Geometry: final body of the model. Coordinates: model frame, mm. A direction names the side the tool comes from. Round coordinates to 2 decimals unless told otherwise and drop trailing zeros. Order: outer loops, then holes, each group sorted by start corner. A loop starts at its lowest first (then second) coordinate and runs counter-clockwise, first axis right, second up. Notation, with made-up numbers: M 70,-36.75 L 121,-36.75 A22 ccw 121,-7.75 Z; hole C -39,85.5 d5. An arc over 180 degrees is marked long. Return JSON: item names as keys, results as strings. Group by question number.
Q1. Ray query, probe 1 along X at (y, z) = (98.5, 4); probe 2 along X at (y, z) = (50.5, 2); probe 3 along Y at (x, z) = (74, 6). Return the intervals inside material, ascending.
Q2. Cut plane A-A on x = 61.5. Output: boundary loops of the cut face in (y, z).
Q3. Contact query for flat-ended pins moving along their axis: pin 1 (5 mm diameter, centred on x = 266, y = 111.5, fed in from -Z); pin 2 (4.5 mm diameter, centred on x = 197, y = 79.5, fed in from +Z); pin 3 (0.6 mm diameter, centred on x = 277, z = 5.5, fed in from -Y). Output: stop coordinate, or through.
Q4. Access query for faces 1 (the face through (11, 90, 4)), 2 (the face through (20, 173, 4)), 3 (the face through (86, 66, 5)). Directions: +Z, -Z, +X, -X, +Y, -Y. A direction counts if a zero-diameter tool reaches every point of the face in a straight line with its end or side. Return the directions, or none.
Q5. Mould query, pull axis X, two halves, no side actions, for faces 4 (the face through (6, 22.5, 4)), 5 (the face through (267.308, 19.363, 3.944)), 6 (the face through (20, 7, 4)), 7 (the face through (76.5, 90, 4)). Classes: released by +X, released by -X, zero draft, split by the parting line, or undercut.
Q6. Cut plane B-B on z = 3. Count the separate pieces of the cut face and the enclosed holes in it, and give its area (3 significant figures).
```python
from build123d import *

# Parameters (mm, degrees)
ESQUISSE1_W                  = 284
ESQUISSE1_H                  = 180
BOSS_EXTRU_1_DEPTH           = 8
ESQUISSE2_W                  = 29
ESQUISSE2_H                  = 60
ESQUISSE2_W_2                = 8
ENL_V_MAT_EXTRU_1_DEPTH      = 9
ESQUISSE3_R                  = 1.65
ENL_V_MAT_EXTRU_2_DEPTH      = 8
ESQUISSE4_W                  = 8
ESQUISSE4_H                  = 90
ESQUISSE4_H_2                = 50
ENL_V_MAT_EXTRU_3_DEPTH      = 3
ESQUISSE5_R                  = 2
ENL_V_MAT_EXTRU_4_DEPTH      = 9
ESQUISSE6_R                  = 3
ENL_V_MAT_EXTRU_5_DEPTH      = 9
ESQUISSE8_W                  = 20
ESQUISSE8_H                  = 22.5
ENL_V_MAT_EXTRU_7_DEPTH      = 9
CONG_1_R                     = 11
ESQUISSE7_R                  = 1.65
ENL_V_MAT_EXTRU_6_DEPTH      = 9
CONG_2_R                     = 3
ESQUISSE9_R                  = 2
ENL_V_MAT_EXTRU_8_DEPTH      = 3
CONG_3_R                     = 3
ESQUISSE10_R                 = 2
ENL_V_MAT_EXTRU_9_DEPTH      = 6
ESQUISSE11_R                 = 2
ESQUISSE11_R_2               = 3
ENL_V_MAT_EXTRU_10_DEPTH     = 9
ESQUISSE12_R                 = 1.75
ENL_V_MAT_EXTRU_11_DEPTH     = 9
ESQUISSE13_R                 = 2
ENL_V_MAT_EXTRU_12_DEPTH     = 9
ESQUISSE14_R                 = 3
FIXATIONS_USINAGE_DEPTH      = 1
FIXATIONS_USINAGE_DEPTH_BACK = 9


with BuildPart() as part:
    # Esquisse1 → Boss.-Extru.1 (new body)
    with BuildSketch(Plane.XY):
        with Locations((142, 90)):
            Rectangle(ESQUISSE1_W, ESQUISSE1_H)
    extrude(amount=BOSS_EXTRU_1_DEPTH)

    # Esquisse2 → Enlèv. mat.-Extru.1 (cut, through all)
    with BuildSketch(Plane.XY.offset(8)):
        with Locations((62, 90)):
            Rectangle(ESQUISSE2_W, ESQUISSE2_H)
        with Locations((7, 90)):
            Rectangle(ESQUISSE2_W_2, ESQUISSE2_H)
        with Locations((277, 90)):
            Rectangle(ESQUISSE2_W_2, ESQUISSE2_H)
        with Locations((222, 90)):
            Rectangle(ESQUISSE2_W, ESQUISSE2_H)
    extrude(amount=-ENL_V_MAT_EXTRU_1_DEPTH, mode=Mode.SUBTRACT)

    # Esquisse3 → Enlèv. mat.-Extru.2 (cut)
    with BuildSketch(Plane.XY.offset(8)):
        with Locations((112, 172)):
            Circle(ESQUISSE3_R)
        with Locations((172, 172)):
            Circle(ESQUISSE3_R)
        with Locations((232, 172)):
            Circle(ESQUISSE3_R)
        with Locations((52, 172)):
            Circle(ESQUISSE3_R)
    extrude(amount=-ENL_V_MAT_EXTRU_2_DEPTH, mode=Mode.SUBTRACT)

    # Esquisse4 → Enlèv. mat.-Extru.3 (cut)
    with BuildSketch(Plane.XY.offset(8)):
        with Locations((88, 65)):
            Rectangle(ESQUISSE4_W, ESQUISSE4_H)
        with Locations((196, 65)):
            Rectangle(ESQUISSE4_W, ESQUISSE4_H)
        with Locations((41.5, 90)):
            Rectangle(ESQUISSE4_W, ESQUISSE4_H_2)
        with Locations((242.5, 90)):
            Rectangle(ESQUISSE4_W, ESQUISSE4_H_2)
    extrude(amount=-ENL_V_MAT_EXTRU_3_DEPTH, mode=Mode.SUBTRACT)

    # Esquisse5 → Enlèv. mat.-Extru.4 (cut, through all)
    with BuildSketch(Plane.XY.offset(8)):
        with Locations((123, 129)):
            Circle(ESQUISSE5_R)
        with Locations((123, 105)):
            Circle(ESQUISSE5_R)
        with Locations((161, 105)):
            Circle(ESQUISSE5_R)
        with Locations((161, 129)):
            Circle(ESQUISSE5_R)
    extrude(amount=-ENL_V_MAT_EXTRU_4_DEPTH, mode=Mode.SUBTRACT)

    # Esquisse6 → Enlèv. mat.-Extru.5 (cut, through all)
    with BuildSketch(Plane.XY.offset(8)):
        with Locations((18, 111.5)):
            Circle(ESQUISSE6_R)
        with Locations((18, 68.5)):
            Circle(ESQUISSE6_R)
        with Locations((266, 68.5)):
            Circle(ESQUISSE6_R)
        with Locations((266, 111.5)):
            Circle(ESQUISSE6_R)
    extrude(amount=-ENL_V_MAT_EXTRU_5_DEPTH, mode=Mode.SUBTRACT)

    # Esquisse8 → Enlèv. mat.-Extru.7 (cut, through all)
    with BuildSketch(Plane.XY.offset(8)):
        with Locations((10, 168.75)):
            Rectangle(ESQUISSE8_W, ESQUISSE8_H)
        with Locations((274, 168.75)):
            Rectangle(ESQUISSE8_W, ESQUISSE8_H)
        with Locations((274, 11.25)):
            Rectangle(ESQUISSE8_W, ESQUISSE8_H)
        with Locations((10, 11.25)):
            Rectangle(ESQUISSE8_W, ESQUISSE8_H)
    extrude(amount=-ENL_V_MAT_EXTRU_7_DEPTH, mode=Mode.SUBTRACT)

    # Congé1
    cong_1_edges = [part.edges().sort_by_distance(p)[0] for p in [
        (20, 157.5, 4),
        (264, 157.5, 4),
        (20, 22.5, 4),
        (264, 22.5, 4),
    ]]
    fillet(cong_1_edges, radius=CONG_1_R)

    # Esquisse7 → Enlèv. mat.-Extru.6 (cut, through all)
    with BuildSketch(Plane.XY.offset(8)):
        with Locations((33, 155)):
            Circle(ESQUISSE7_R)
        with Locations((23.473720558, 160.5)):
            Circle(ESQUISSE7_R)
        with Locations((260.526279442, 160.5)):
            Circle(ESQUISSE7_R)
        with Locations((251, 155)):
            Circle(ESQUISSE7_R)
        with Locations((23.473720558, 19.5)):
            Circle(ESQUISSE7_R)
        with Locations((33, 25)):
            Circle(ESQUISSE7_R)
        with Locations((251, 25)):
            Circle(ESQUISSE7_R)
        with Locations((260.526279442, 19.5)):
            Circle(ESQUISSE7_R)
    extrude(amount=-ENL_V_MAT_EXTRU_6_DEPTH, mode=Mode.SUBTRACT)

    # Congé2
    cong_2_edges = [part.edges().sort_by_distance(p)[0] for p in [
        (47.5, 60, 4),
        (47.5, 120, 4),
        (76.5, 120, 4),
        (76.5, 60, 4),
        (3, 60, 4),
        (3, 120, 4),
        (11, 120, 4),
        (11, 60, 4),
        (281, 60, 4),
        (273, 60, 4),
        (273, 120, 4),
        (281, 120, 4),
        (236.5, 60, 4),
        (207.5, 60, 4),
        (207.5, 120, 4),
        (236.5, 120, 4),
    ]]
    fillet(cong_2_edges, radius=CONG_2_R)

    # Esquisse9 → Enlèv. mat.-Extru.8 (cut)
    with BuildSketch(Plane.XY.offset(8)):
        with Locations((38.843502884, 113.656497116)):
            Circle(ESQUISSE9_R)
        with Locations((44.156497116, 113.656497116)):
            Circle(ESQUISSE9_R)
        with Locations((44.156497116, 66.343502884)):
            Circle(ESQUISSE9_R)
        with Locations((38.843502884, 66.343502884)):
            Circle(ESQUISSE9_R)
        with Locations((245.156497116, 66.343502884)):
            Circle(ESQUISSE9_R)
        with Locations((239.843502884, 66.343502884)):
            Circle(ESQUISSE9_R)
        with Locations((239.843502884, 113.656497116)):
            Circle(ESQUISSE9_R)
        with Locations((245.156497116, 113.656497116)):
            Circle(ESQUISSE9_R)
        with Locations((85.343502884, 108.656497116)):
            Circle(ESQUISSE9_R)
        with Locations((90.656497116, 108.656497116)):
            Circle(ESQUISSE9_R)
        with Locations((90.656497116, 21.343502884)):
            Circle(ESQUISSE9_R)
        with Locations((85.343502884, 21.343502884)):
            Circle(ESQUISSE9_R)
        with Locations((198.656497116, 21.343502884)):
            Circle(ESQUISSE9_R)
        with Locations((193.343502884, 21.343502884)):
            Circle(ESQUISSE9_R)
        with Locations((193.343502884, 108.656497116)):
            Circle(ESQUISSE9_R)
        with Locations((198.656497116, 108.656497116)):
            Circle(ESQUISSE9_R)
    extrude(amount=-ENL_V_MAT_EXTRU_8_DEPTH, mode=Mode.SUBTRACT)

    # Congé3
    cong_3_edges = [part.edges().sort_by_distance(p)[0] for p in [
        (0, 157.5, 4),
        (20, 180, 4),
        (264, 180, 4),
        (284, 157.5, 4),
        (0, 22.5, 4),
        (20, 0, 4),
        (264, 0, 4),
        (284, 22.5, 4),
    ]]
    fillet(cong_3_edges, radius=CONG_3_R)

    # Esquisse10 → Enlèv. mat.-Extru.9 (cut, through all)
    with BuildSketch(Plane.XY.offset(5)):
        with Locations((41.5, 90)):
            Circle(ESQUISSE10_R)
        with Locations((41.5, 70)):
            Circle(ESQUISSE10_R)
        with Locations((41.5, 110)):
            Circle(ESQUISSE10_R)
        with Locations((88, 65)):
            Circle(ESQUISSE10_R)
        with Locations((88, 25)):
            Circle(ESQUISSE10_R)
        with Locations((88, 105)):
            Circle(ESQUISSE10_R)
        with Locations((196, 105)):
            Circle(ESQUISSE10_R)
        with Locations((196, 25)):
            Circle(ESQUISSE10_R)
        with Locations((196, 65)):
            Circle(ESQUISSE10_R)
        with Locations((242.5, 110)):
            Circle(ESQUISSE10_R)
        with Locations((242.5, 70)):
            Circle(ESQUISSE10_R)
        with Locations((242.5, 90)):
            Circle(ESQUISSE10_R)
    extrude(amount=-ENL_V_MAT_EXTRU_9_DEPTH, mode=Mode.SUBTRACT)

    # Esquisse11 → Enlèv. mat.-Extru.10 (cut, through all)
    with BuildSketch(Plane.XY.offset(8)):
        with Locations((47, 16)):
            Circle(ESQUISSE11_R)
        with Locations((237, 16)):
            Circle(ESQUISSE11_R)
        with Locations((102, 16)):
            Circle(ESQUISSE11_R)
        with Locations((46.5, 26)):
            Circle(ESQUISSE11_R_2)
        with Locations((54.5, 26)):
            Circle(ESQUISSE11_R_2)
        with Locations((229.5, 26)):
            Circle(ESQUISSE11_R_2)
        with Locations((237.5, 26)):
            Circle(ESQUISSE11_R_2)
        with Locations((182, 16)):
            Circle(ESQUISSE11_R)
    extrude(amount=-ENL_V_MAT_EXTRU_10_DEPTH, mode=Mode.SUBTRACT)

    # Esquisse12 → Enlèv. mat.-Extru.11 (cut, through all)
    with BuildSketch(Plane.XY.offset(8)):
        with Locations((128, 4)):
            Circle(ESQUISSE12_R)
        with Locations((128, 19)):
            Circle(ESQUISSE12_R)
    extrude(amount=-ENL_V_MAT_EXTRU_11_DEPTH, mode=Mode.SUBTRACT)

    # Esquisse13 → Enlèv. mat.-Extru.12 (cut, through all)
    with BuildSketch(Plane.XY.offset(8)):
        with Locations((4, 30)):
            Circle(ESQUISSE13_R)
        with Locations((4, 50)):
            Circle(ESQUISSE13_R)
        with Locations((4, 130)):
            Circle(ESQUISSE13_R)
        with Locations((4, 150)):
            Circle(ESQUISSE13_R)
        with Locations((280, 150)):
            Circle(ESQUISSE13_R)
        with Locations((280, 130)):
            Circle(ESQUISSE13_R)
        with Locations((280, 50)):
            Circle(ESQUISSE13_R)
        with Locations((280, 30)):
            Circle(ESQUISSE13_R)
    extrude(amount=-ENL_V_MAT_EXTRU_12_DEPTH, mode=Mode.SUBTRACT)

    # Esquisse14 → fixations_usinage (cut, two sides)
    with BuildSketch(Plane.XY.offset(8)) as fixations_usinage_sk:
        with Locations((42, 140)):
            Circle(ESQUISSE14_R)
        with Locations((42, 40)):
            Circle(ESQUISSE14_R)
        with Locations((242, 40)):
            Circle(ESQUISSE14_R)
        with Locations((242, 140)):
            Circle(ESQUISSE14_R)
        with Locations((142, 40)):
            Circle(ESQUISSE14_R)
        with Locations((142, 140)):
            Circle(ESQUISSE14_R)
    extrude(amount=FIXATIONS_USINAGE_DEPTH, mode=Mode.SUBTRACT)
    extrude(fixations_usinage_sk.sketch, amount=-FIXATIONS_USINAGE_DEPTH_BACK, mode=Mode.SUBTRACT)


solid = part.part
```
Result sheet:
{
 "1": {"probe 1": "x = 0 to 3, 11 to 47.5, 76.5 to 207.5, 236.5 to 273, 281 to 284", "probe 2": "x = 0 to 2.06, 5.94 to 278.06, 281.94 to 284", "probe 3": "y = 0 to 60.04, 119.96 to 180"},
 "2": {"outline": "M 0,0 L 60,0 L 60,8 L 0,8 Z; M 120,0 L 180,0 L 180,8 L 120,8 Z"},
 "3": {"pin 1": "passes through", "pin 2": "stops at z = 5", "pin 3": "stops at y = 22.5"},
 "4": {"face 1": "+Z, -Z", "face 2": "+Z, -Z, -X, +Y", "face 3": "+Z"},
 "5": {"face 4": "zero draft", "face 5": "released by +X", "face 6": "released by -X", "face 7": "undercut"},
 "6": {"separate pieces": "1", "enclosed holes": "60", "area": "44,100 mm²"}
}
